Design review of the part shown in the three views and the two pictorial views. Dimensions are in mm from the part's minimum x, y and z. A direction names the side the tool comes from. Give positions to 0.01 mm unless a question says otherwise; leave off trailing zeros. Loops run counter-clockwise (first coordinate to the right, second up) from the corner with the lowest first, then second, coordinate; pieces in that order, holes last. Notation, with made-up numbers: (27.5, 9.5) - (54.5, 9.5) arc R30 ccw to (54.5, 45.5) - close; hole circle Ø6 at (-21, 43). An arc over 180 degrees is marked (long way). Put each result on its own line as item: value. Start each with the question number.
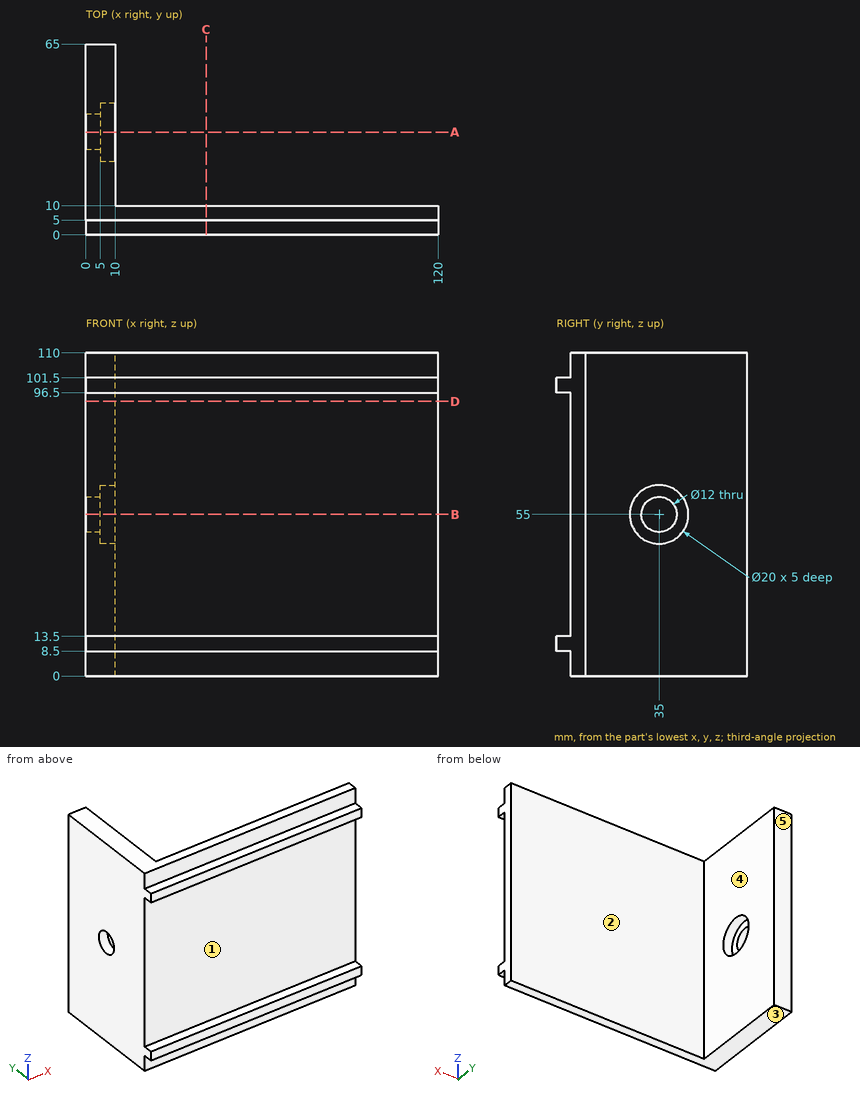
1) Machinability: for the marked faces 4 and 5, which of the approach directions +Z, -Z, +X, -X, +Y, -Y give a long, thin tool a straight path to every point of the face, cutting with its end or side? Answer none if there is none.
2) Take a section at C-C on x = 41. State the section outline as (y, z) points.
3) Take a section at A-A on y = 35. State the section outline as (x, z) points.
4) Take a section at B-B on z = 55. State the section outline as (x, y) points, and give its area (3 significant figures).
5) Insertion check: P1, Ø2, axis at x = 45.5, z = 34, coming from the +Y side; P2, Ø4, axis at x = 36.5, z = 107.5, coming from the -Y side; P3, Ø3, axis at y = 51, z = 91, coming from the +X side. Each pin has a flat end and moves straight along its axis. Give the tip position at first contact, or say it passes through.
6) Mouldability with a two-part tool opening along Z and no side actions: class the marked faces 1, 2 and 3 as released by +Z, released by -Z, zero draft, split by the parting line, or undercut.
7) Wall thickness on probe 1 along Y at (x, z) = (2, 55); probe 2 along X at (y, z) = (27, 61.5): over which ranges is each line inside the solid? List them lowest first.
8) Take a section at D-D on z = 93.5. State the section outline as (x, y) points.
Answers follow:
1. face 4: +Z, -Z, +X, +Y
1. face 5: +Z, -Z, +X, -X, +Y
2. outline: (0, 8.5) - (5, 8.5) - (5, 0) - (10, 0) - (10, 110) - (5, 110) - (5, 101.5) - (0, 101.5) - (0, 96.5) - (5, 96.5) - (5, 13.5) - (0, 13.5) - close
3. outline: (0, 0) - (10, 0) - (10, 45) - (5, 45) - (5, 49) - (0, 49) - close; (0, 61) - (5, 61) - (5, 65) - (10, 65) - (10, 110) - (0, 110) - close
4. outline: (0, 5) - (120, 5) - (120, 10) - (10, 10) - (10, 25) - (5, 25) - (5, 29) - (0, 29) - close; (0, 41) - (5, 41) - (5, 45) - (10, 45) - (10, 65) - (0, 65) - close
4. area: 990 mm2
5. P1: y = 10
5. P2: y = 5
5. P3: x = 10
6. face 1: undercut
6. face 2: zero draft
6. face 3: released by -Z
7. probe 1: 5 to 29, 41 to 65
7. probe 2: 0 to 10
8. outline: (0, 5) - (120, 5) - (120, 10) - (10, 10) - (10, 65) - (0, 65) - close
